Autodesk Inventor part; units mm, degrees
ref_plane "YZ Plane" through (0, 0, 0) normal (1, 0, 0) x (0, 1, 0)
ref_plane "XZ Plane" through (0, 0, 0) normal (0, 1, 0) x (-1, 0, 0)
ref_plane "XY Plane" through (0, 0, 0) normal (0, 0, 1) x (1, 0, 0)
sketch "Skizze1" plane through (0, 0, 0) normal (0, 1, 0) x (-1, 0, 0)
  circle A0 centre (-44.3776, -92.6293) radius 1.6
  circle A1 centre (92.6293, 44.3776) radius 1.6
  circle A2 centre (-92.6293, -44.3776) radius 1.6
  circle A3 centre (44.3776, -92.6293) radius 1.6
  circle A4 centre (92.6293, -44.3776) radius 1.6
  circle A5 centre (-92.6293, 44.3776) radius 1.6
  circle A6 centre (45, 91.781) radius 1.6
  circle A7 centre (-45, 91.781) radius 1.6
  arc A8 (12, 71.7738) -> (39.8653, 97.0306) centre (12, 99.7738) ccw
  line L0 (-12, 71.7738) -> (12, 71.7738)
  arc A9 (-39.8653, 97.0306) -> (-12, 71.7738) centre (-12, 99.7738) ccw
  arc A10 (-39.8653, 97.0306) -> (-42.6492, 98.6705) centre (-41.8557, 96.8347) ccw
  arc A11 (-42.6492, 98.6705) -> (-50.5184, 94.8829) centre (0, -0.0072) ccw
  arc A12 (-50.5184, 94.8829) -> (-51.2299, 90.1135) centre (-49.1086, 92.2348) ccw
  line L1 (-49.4975, 88.3811) -> (-51.2299, 90.1135)
  arc A13 (-49.4975, 74.239) -> (-49.4975, 88.3811) centre (-56.5685, 81.31) ccw
  line L2 (-74.2462, 49.4902) -> (-49.4975, 74.239)
  arc A14 (-88.3883, 49.4902) -> (-74.2462, 49.4902) centre (-81.3173, 56.5613) ccw
  line L3 (-90.1208, 51.2226) -> (-88.3883, 49.4902)
  arc A15 (-90.1208, 51.2226) -> (-94.8902, 50.5111) centre (-92.2421, 49.1013) ccw
  arc A16 (-94.8902, 50.5111) -> (-94.8902, -50.5256) centre (0, -0.0072) ccw
  arc A17 (-94.8902, -50.5256) -> (-90.1207, -51.2371) centre (-92.2421, -49.1158) ccw
  line L4 (-88.3883, -49.5047) -> (-90.1207, -51.2371)
  arc A18 (-74.2462, -49.5047) -> (-88.3883, -49.5047) centre (-81.3173, -56.5758) ccw
  line L5 (-49.4975, -74.2535) -> (-74.2462, -49.5047)
  arc A19 (-49.4975, -88.3956) -> (-49.4975, -74.2535) centre (-56.5685, -81.3245) ccw
  line L6 (-51.2299, -90.128) -> (-49.4975, -88.3956)
  arc A20 (-51.2299, -90.128) -> (-50.5184, -94.8974) centre (-49.1086, -92.2493) ccw
  arc A21 (-50.5184, -94.8974) -> (50.5184, -94.8974) centre (0, -0.0072) ccw
  arc A22 (50.5184, -94.8974) -> (51.2299, -90.128) centre (49.1086, -92.2493) ccw
  line L7 (49.4975, -88.3956) -> (51.2299, -90.128)
  arc A23 (49.4975, -74.2535) -> (49.4975, -88.3956) centre (56.5685, -81.3245) ccw
  line L8 (74.2462, -49.5047) -> (49.4975, -74.2535)
  arc A24 (88.3883, -49.5047) -> (74.2462, -49.5047) centre (81.3173, -56.5758) ccw
  line L9 (90.1208, -51.2371) -> (88.3883, -49.5047)
  arc A25 (90.1208, -51.2371) -> (94.8902, -50.5256) centre (92.2421, -49.1158) ccw
  arc A26 (94.8902, -50.5256) -> (94.8902, 50.5111) centre (0, -0.0072) ccw
  arc A27 (94.8902, 50.5111) -> (90.1207, 51.2226) centre (92.2421, 49.1013) ccw
  line L10 (88.3883, 49.4902) -> (90.1207, 51.2226)
  arc A28 (74.2462, 49.4902) -> (88.3883, 49.4902) centre (81.3173, 56.5613) ccw
  line L11 (49.4975, 74.239) -> (74.2462, 49.4902)
  arc A29 (49.4975, 88.3811) -> (49.4975, 74.239) centre (56.5685, 81.31) ccw
  line L12 (51.2299, 90.1135) -> (49.4975, 88.3811)
  arc A30 (51.2299, 90.1135) -> (50.5184, 94.8829) centre (49.1086, 92.2348) ccw
  arc A31 (50.5184, 94.8829) -> (42.6492, 98.6705) centre (0, -0.0072) ccw
  arc A32 (42.6492, 98.6705) -> (39.8653, 97.0306) centre (41.8557, 96.8347) ccw
  circle A33 centre (-48.7904, 67.8822) radius 1.6
  circle A34 centre (48.7904, 67.8823) radius 1.6
  circle A35 centre (67.8822, 48.7904) radius 1.6
  circle A36 centre (-67.8823, 48.7904) radius 1.6
  circle A37 centre (67.8823, -48.7904) radius 1.6
  circle A38 centre (48.7904, -67.8822) radius 1.6
  circle A39 centre (-48.7904, -67.8823) radius 1.6
  circle A40 centre (-67.8822, -48.7904) radius 1.6
  arc A41 (-83.3481, 25.2693) -> (-60.278, 34.4345) centre (-81.8968, 55.2341) ccw
  arc A42 (-58.8889, -36.4356) -> (-82.2957, -28.1679) centre (-79.6885, -58.0544) ccw
  line L13 (-58.8889, -36.4356) -> (-49.1604, -45.7954)
  line L14 (-49.1604, -45.7954) -> (-43.3954, -51.342)
  line L15 (-43.3954, -51.342) -> (-33.6669, -60.7018)
  arc A43 (-24.5017, -83.772) -> (-33.6669, -60.7018) centre (-54.4666, -82.3207) ccw
  arc A44 (37.0306, -59.3366) -> (28.7629, -82.7434) centre (58.6494, -80.1363) ccw
  line L16 (37.0306, -59.3366) -> (46.3904, -49.6081)
  line L17 (46.3904, -49.6081) -> (51.937, -43.8431)
  line L18 (51.937, -43.8431) -> (61.2969, -34.1146)
  arc A45 (83.8457, -25.0231) -> (61.2969, -34.1146) centre (82.8273, -55.0058) ccw
  arc A46 (60.905, 36.457) -> (82.8171, 28.2415) centre (81.5589, 58.2151) ccw
  line L19 (60.905, 36.457) -> (51.1766, 45.8169)
  line L20 (51.1766, 45.8169) -> (45.4116, 51.3634)
  line L21 (45.4116, 51.3634) -> (37.2169, 59.4013)
  arc A47 (12.5, 52.2686) -> (37.2169, 59.4013) centre (12.0366, 100.2664) ccw
  line L22 (-12.47, 51.7864) -> (-12.5, 51.7858)
  arc A48 (-37.4131, 58.1998) -> (-12.5, 51.7858) centre (-13.4268, 99.7769) ccw
  line L23 (-37.4131, 58.1998) -> (-45.3715, 49.9279)
  line L24 (-45.3715, 49.9279) -> (-50.9181, 44.1629)
  line L25 (-50.9181, 44.1629) -> (-60.278, 34.4345)
  line L26 (12.5, 12.4928) -> (12.5, 52.2686)
  line L27 (-12.5, 12.4928) -> (-12.5, 51.7858)
  line L28 (12.5, -12.5072) -> (86.6015, -12.5072)
  line L29 (12.5, 12.4928) -> (86.6036, 12.4928)
  line L30 (12.5, -12.5072) -> (12.5, -86.6025)
  line L31 (-12.5, -12.5072) -> (-12.5, -86.452)
  line L32 (-12.5, -12.5072) -> (-86.0925, -12.5072)
  line L33 (-12.4928, 12.4928) -> (-86.1498, 12.4928)
  arc A49 (-83.3481, 25.2693) -> (-86.1498, 12.4928) centre (0.4811, 0.1913) ccw
  arc A50 (-86.0925, -12.5072) -> (-82.2957, -28.1679) centre (0.4811, 0.1913) ccw
  arc A51 (83.8457, -25.0231) -> (86.6015, -12.5072) centre (0, 0) ccw
  arc A52 (86.6036, 12.4928) -> (82.8171, 28.2415) centre (0, 0) ccw
  arc A53 (-24.5017, -83.772) -> (-12.5, -86.452) centre (0.5214, 0.0737) ccw
  arc A54 (12.5, -86.6025) -> (28.7629, -82.7434) centre (0.5214, 0.0737) ccw
extrude "Extrusion1" add sketch "Skizze1" along normal blind 2
properties part number "Boden WM"
CAD build for the part. Positions are in the model's coordinates, mm. A direction names the side the tool comes from. Coordinates: 2 decimals unless noted, no trailing zeros. Order: outer loops, then holes, each group sorted by start corner. A loop starts at its lowest first (then second) coordinate and runs counter-clockwise, first axis right, second up. Notation, with made-up numbers: M 23,-8 L 74,-8 A8 ccw 74,6 Z; hole C 61.5,27.5 d10. An arc over 180 degrees is marked long. Write each question's results on one line, items separated by ' | '. Start each with the question number.
Q1. Cut at A-A (z = -78). List the corners of the cut face in (x, y).
Q2. Cut at C-C (y = 0.95). Count the separate pieces of the cut face and the enclosed holes in it, then the cut area to 3 significant figures.
Q3. Flat gauge pins, fed straight in: P1, Ø10, axis at x = 66.5, z = 7.5, coming from the -Y side; P2, Ø1.9, axis at x = 92.63, z = -44.38, coming from the -Y side; P3, Ø1, axis at y = 0.5, z = 37, coming from the -X side; P4, Ø0.6, axis at x = -43.5, y = 1, coming from the -Z side. Where does each tip first touch, or does it go through?
Q4. Which spindle directions (+Z, -Z, +X, -X, +Y, -Y) get a long thin tool onto all of the face, cutting with end or side? Do faces 1 (the cylindrical face through (26.65, 0.99, -71.08)), 2 (the cylindrical face through (-107.498, 0.986, 0.729)), 3 (the cylindrical face through (30.589, 0.986, 78.835)). Say none if no direction does.
Q5. Drill centre lines: probe 1 along Z at (x, y) = (45, 1.3); probe 2 along X at (y, z) = (0.1, -78.5); probe 3 along Z at (x, y) = (60, 1.35). Where is each one in solid material? Low to high. Write a range as from..to.
Q6. Pull direction Z, two halves, no side cores. Call faces 4 (the cylindrical face through (107.497, 0.986, -0.744)), 5 (the cylindrical face through (-30.303, 0.986, -70.314)), 6 (the cylindrical face through (-0.736, 0.986, -107.505)): +Z half, -Z half, draft (parallel to the pull), parting line (faces both ways), or undercut.
Q7. Cut at B-B (x = -19). List the corners of the cut face in (y, z), then the cut area to 3 significant figures.
Found:
1) outline: M -47.14,0 L -28.73,0 L -28.73,2 L -47.14,2 Z; M -12.5,0 L 12.5,0 L 12.5,2 L -12.5,2 Z; M 24.78,0 L 47.14,0 L 47.14,2 L 24.78,2 Z
2) separate pieces: 1 | enclosed holes: 20 | area: 19,800 mm²
3) P1: y = 0 | P2: through | P3: x = -101.11 | P4: z = -98.45
4) face 1: +Y, -Y | face 2: -X, +Y, -Y | face 3: +Z, +Y, -Y
5) probe 1: -97.64..-94.1, -91.16..-49.8, -12.51..12.49, 50.31..90.18, 93.38..97.62 | probe 2: -46.98..-28.69, -12.5..12.5, 24.71..46.98 | probe 3: -63.75..-35.42, -12.51..12.49, 34.72..63.74
6) face 4: parting line | face 5: undercut | face 6: -Z half
7) outline: M 0,-105.81 L 2,-105.81 L 2,-85.45 L 0,-85.45 Z; M 0,-12.51 L 2,-12.51 L 2,12.49 L 0,12.49 Z; M 0,52.77 L 2,52.77 L 2,72.66 L 0,72.66 Z | area: 131 mm²
